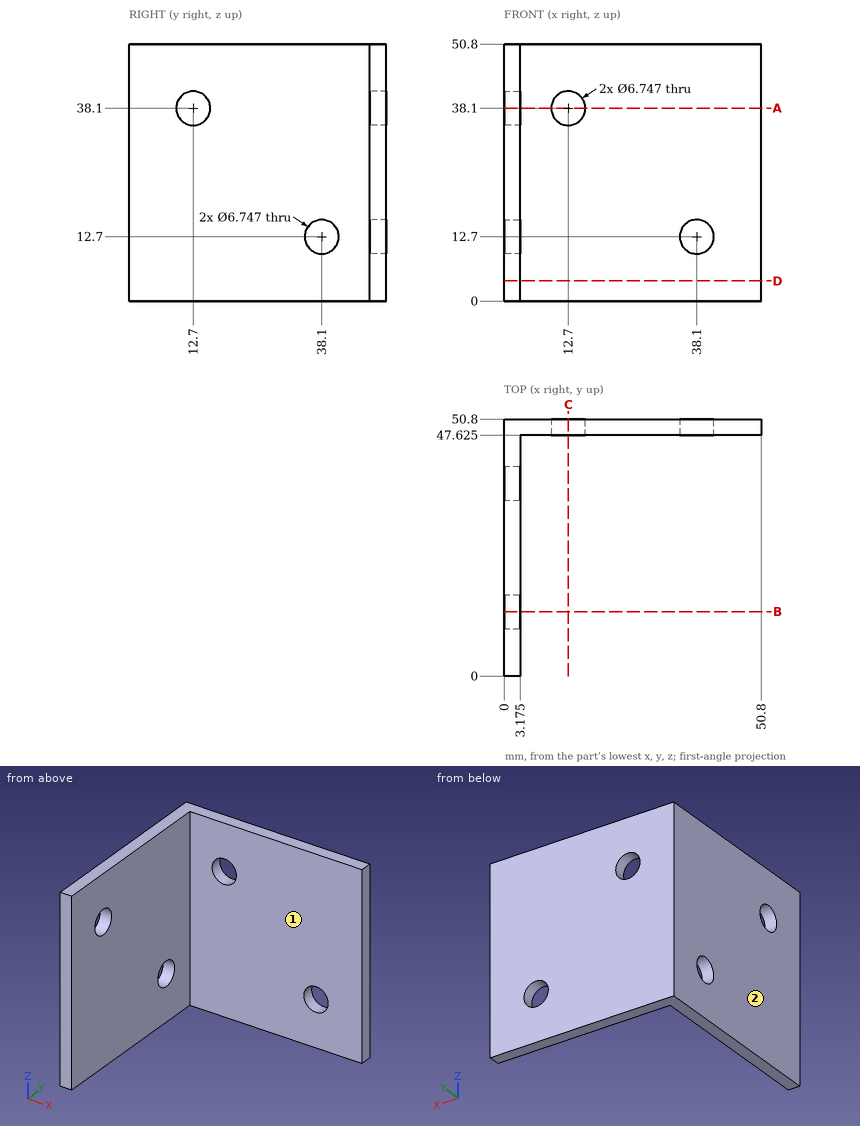
Verification items for this drawing (mm, ordinates from the low corner). A direction names the side the tool comes from. Coordinates: 2 decimals unless noted, no trailing zeros. Loops run counter-clockwise (first coordinate to the right, second up) from the corner with the lowest first, then second, coordinate; pieces in that order, holes last. Notation, with made-up numbers: (39, 61) -> (70, 61) arc R36 cw to (70, 95) -> close; hole circle Ø6 at (51.25, 67.25). An arc over 180 degrees is marked (long way). Put each result on its own line as item: value.
1. Tool access check on the marked faces 1 and 2. Record the directions out of +Z, -Z, +X, -X, +Y, -Y that give a thin tool (end or side, any length) a straight path to the whole face; none if there is none.
Result set:
face 1: +Z, -Z, +X, -Y
face 2: +Z, -Z, -X, +Y, -Y
2. Thickness scan on line 1 (Z direction, x = 12.7, y = 48.4); line 2 (Y direction, x = 35, z = 38) (3 decimals); line 3 (X direction, y = 25, z = 44) (3 decimals). Record the ranges inside material, lowest first.
Result set:
line 1: z = 0 to 34.73, 41.47 to 50.8
line 2: y = 47.625 to 50.8
line 3: x = 0 to 3.175
3. Section check D-D, the plane z = 4. Record the boundary of the cut face in (x, y) (3 decimals).
Result set:
outline: (0, 0) -> (3.175, 0) -> (3.175, 47.625) -> (50.8, 47.625) -> (50.8, 50.8) -> (0, 50.8) -> close
4. Section check B-B, the plane y = 12.7. Record the boundary of the cut face in (x, z) (1 decimal), then the cut area to 3 significant figures.
Result set:
outline: (0, 0) -> (3.2, 0) -> (3.2, 34.7) -> (0, 34.7) -> close; (0, 41.5) -> (3.2, 41.5) -> (3.2, 50.8) -> (0, 50.8) -> close
area: 140 mm^2
5. Section check C-C, the plane x = 12.7. Record the boundary of the cut face in (y, z) (1 decimal).
Result set:
outline: (47.6, 0) -> (50.8, 0) -> (50.8, 34.7) -> (47.6, 34.7) -> close; (47.6, 41.5) -> (50.8, 41.5) -> (50.8, 50.8) -> (47.6, 50.8) -> close
6. Gauge pin test, flat ends, axial feed: P1, Ø2, axis at y = 10.5, z = 33, coming from the +X side (3 decimals); P2, Ø5.5, axis at y = 12.7, z = 38.1, coming from the -X side; P3, Ø1.5, axis at x = 31, z = 18.5, coming from the -Y side (3 decimals). Record the tip position at first contact, or that the pin passes through.
Result set:
P1: stops at x = 3.175
P2: passes through
P3: stops at y = 47.625
7. Section check A-A, the plane z = 38.1. Record the boundary of the cut face in (x, y) (1 decimal), then the cut area to 3 significant figures.
Result set:
outline: (0, 0) -> (3.2, 0) -> (3.2, 9.3) -> (0, 9.3) -> close; (0, 16.1) -> (3.2, 16.1) -> (3.2, 47.6) -> (9.3, 47.6) -> (9.3, 50.8) -> (0, 50.8) -> close; (16.1, 47.6) -> (50.8, 47.6) -> (50.8, 50.8) -> (16.1, 50.8) -> close
area: 270 mm^2
